Work out the finished part from the listing and answer in its coordinate system (mm). A direction names the side the tool comes from. Round coordinates to 2 decimals unless told otherwise and drop trailing zeros. Write each loop counter-clockwise with the first axis right and the second up, starting at its lowest first coordinate (ties: lowest second). Pieces come first, ordered by that corner, then holes. Notation, with made-up numbers: (19, 37) -> (58, 37) arc R20 cw to (58, 73) -> close; hole circle Ø9 at (-10.5, 39.25). An arc over 180 degrees is marked (long way). One line per item, written item: value.
```python
from build123d import *

# Parameters (mm, degrees)
MODEL_R                 = 8
MODEL_R_2               = 6
MODEL_W                 = 24.38
MODEL_H                 = 7.58
SALIENTE_EXTRUIR1_DEPTH = 3


with BuildPart() as part:
    # Model → Saliente-Extruir1 (new body)
    with BuildSketch(Plane.XY):
        with BuildLine():
            Line((11, -3), (21, -3))
            Line((21, -3), (21, 0))
            Line((21, 0), (39, 0))
            Line((39, 0), (39, -3))
            Line((39, -3), (49, -3))
            Line((49, -3), (49, 0))
            Line((49, 0), (60, 0))
            Line((60, 0), (60, 64.525075061))
            ThreePointArc((60, 64.525075061), (59.367904368, 65.768881419), (58.24156757, 66.592267452))
            ThreePointArc((58.24156757, 66.592267452), (52.456145593, 70.630164346), (50.622765109, 77.442978358))
            ThreePointArc((50.622765109, 77.442978358), (41.429140717, 75.658422531), (33.342205195, 70.935198758))
            ThreePointArc((33.342205195, 70.935198758), (29.382797484, 74.208773689), (27.305382782, 78.907449077))
            ThreePointArc((27.305382782, 78.907449077), (21.957335965, 76.972641815), (17.379828576, 73.597510706))
            ThreePointArc((17.379828576, 73.597510706), (16.332778743, 76.092709519), (17.356774707, 78.597457558))
            ThreePointArc((17.356774707, 78.597457558), (10.717974601, 76.180887797), (5.38917768, 71.542202679))
            ThreePointArc((5.38917768, 71.542202679), (4.894477072, 74.219269154), (5.536201967, 76.864945392))
            ThreePointArc((5.536201967, 76.864945392), (1.487784828, 72.953916782), (0, 67.525075061))
            Line((0, 67.525075061), (0, 57.374648319))
            Line((0, 57.374648319), (0, 33.26253753))
            Line((0, 33.26253753), (0, 11.520097779))
            Line((0, 11.520097779), (0, 0))
            Line((0, 0), (11, 0))
            Line((11, 0), (11, -3))
        make_face()
        with Locations((43, 54.525075061)):
            Circle(MODEL_R, mode=Mode.SUBTRACT)
        with Locations((17, 54.525075061)):
            Circle(MODEL_R, mode=Mode.SUBTRACT)
        with Locations((30, 34.525075061)):
            Circle(MODEL_R_2, mode=Mode.SUBTRACT)
        with Locations((30, 13.609080994)):
            Rectangle(MODEL_W, MODEL_H, mode=Mode.SUBTRACT)
    extrude(amount=SALIENTE_EXTRUIR1_DEPTH)


solid = part.part
```
(1) Consider probe 1 along X at (y, z) = (55, 0.6); probe 2 along X at (y, z) = (17, 2.8); probe 3 along X at (y, z) = (73, 0.25). Determine where each line is inside the solid, lowest interval first.
Reported:
probe 1: x = 0 to 9.01, 24.99 to 35.01, 50.99 to 60
probe 2: x = 0 to 17.81, 42.19 to 60
probe 3: x = 1.52 to 4.98, 6.67 to 30.44, 36.15 to 51.22
(2) Find section B-B on y = 38. Give the vertices of the cut face in (x, z).
Reported:
outline: (0, 0) -> (25.11, 0) -> (25.11, 3) -> (0, 3) -> close; (34.89, 0) -> (60, 0) -> (60, 3) -> (34.89, 3) -> close
(3) Find section A-A on x = 15.5. Give the vertices of the cut face in (y, z).
Reported:
outline: (-3, 0) -> (46.67, 0) -> (46.67, 3) -> (-3, 3) -> close; (62.38, 0) -> (78.19, 0) -> (78.19, 3) -> (62.38, 3) -> close
(4) For a pull along X with two mould halves and no side action, classify faces 1 (the face through (29.43, 74.15, 1.48)), 2 (the face through (23, 39, 3)), 3 (the face through (11, -1, 1)), 4 (the face through (52.514, 70.548, 1.479)) as pulls with the +X half, pulls with the -X half, needs draft (parallel to the pull), parting line crosses it, or undercut.
Reported:
face 1: undercut
face 2: needs draft
face 3: pulls with the -X half
face 4: pulls with the +X half
(5) Flat-ended cylindrical pins translate along their axes: pin 1 Ø6 at (x, y) = (18.5, 6.5) entering from -Z; pin 2 Ø0.9 at (x, z) = (5, 1) entering from -Y; pin 3 Ø1 at (x, z) = (17.5, 1) entering from +Y; pin 4 Ø9.5 at (x, y) = (17, 54.53) entering from -Z. Find the tip coordinate at first contact, or state that the pin passes through.
Reported:
pin 1: stops at z = 0
pin 2: stops at y = 0
pin 3: stops at y = 78.6
pin 4: passes through
(6) A tool of negligible diameter and unlimited length cuts with its end or side. For faces 5 (the face through (30, 17.399, 1)), 6 (the face through (49, -2, 1)), 7 (the face through (41.553, 75.705, 1.479)), from which of +Z, -Z, +X, -X, +Y, -Y can it reach the whole face along a straight path? Write none if from no direction.
Reported:
face 5: +Z, -Z
face 6: +Z, -Z, +X, -Y
face 7: +Z, -Z, +Y
(7) Find section C-C on x = 32. Give the vertices of the cut face in (y, z), plus the area to 3 significant figures.
Reported:
outline: (0, 0) -> (9.82, 0) -> (9.82, 3) -> (0, 3) -> close; (17.4, 0) -> (28.87, 0) -> (28.87, 3) -> (17.4, 3) -> close; (40.18, 0) -> (71.72, 0) -> (71.72, 3) -> (40.18, 3) -> close
area: 158 mm2
(8) Find section D-D on z = 2.45. Give the vertices of the cut face in (x, y).
Reported:
outline: (0, 0) -> (11, 0) -> (11, -3) -> (21, -3) -> (21, 0) -> (39, 0) -> (39, -3) -> (49, -3) -> (49, 0) -> (60, 0) -> (60, 64.53) arc R3 ccw to (58.24, 66.59) arc R10.31 cw to (50.62, 77.44) arc R27.93 ccw to (33.34, 70.94) arc R11.18 cw to (27.31, 78.91) arc R19.8 ccw to (17.38, 73.6) arc R3.54 cw to (17.36, 78.6) arc R19.35 ccw to (5.39, 71.54) arc R6.52 cw to (5.54, 76.86) arc R10.64 ccw to (0, 67.53) -> close; hole circle Ø16 at (17, 54.53); hole (17.81, 9.82) -> (42.19, 9.82) -> (42.19, 17.4) -> (17.81, 17.4) -> close; hole circle Ø12 at (30, 34.53); hole circle Ø16 at (43, 54.53)
